Here's the drawing with two shaded views (mm, measured from the low corner). I have some questions. A direction names the side the tool comes from. Round coordinates to 2 decimals unless told otherwise and drop trailing zeros. Loops run counter-clockwise (first coordinate to the right, second up) from the corner with the lowest first, then second, coordinate; pieces in that order, holes last. Notation, with made-up numbers: (10, 26.25) - (38, 26.25) arc R28 cw to (38, 52.25) - close; hole circle Ø11 at (52, 64.25). An arc over 180 degrees is marked (long way). Answer as CSV lines item,"result".
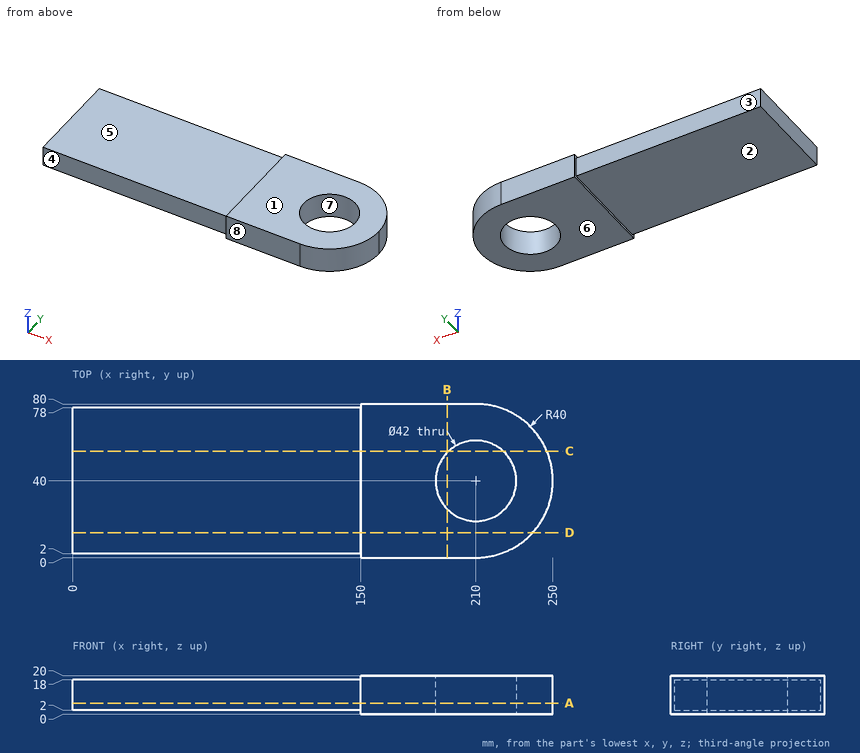
Q1. Imagine slicing it at D-D (y = 13). Write out the boundary of the cut face in (x, z).
Checks:
outline,"(0, 2) - (150, 2) - (150, 0) - (239.51, 0) - (239.51, 20) - (150, 20) - (150, 18) - (0, 18) - close"
Q2. Imagine slicing it at B-B (x = 195). Write out the boundary of the cut face in (y, z).
Checks:
outline,"(0, 0) - (25.3, 0) - (25.3, 20) - (0, 20) - close; (54.7, 0) - (80, 0) - (80, 20) - (54.7, 20) - close"
Q3. Imagine slicing it at C-C (y = 55.5). Write out the boundary of the cut face in (x, z), then the cut area to 3 significant figures.
Checks:
outline,"(0, 2) - (150, 2) - (150, 0) - (195.83, 0) - (195.83, 20) - (150, 20) - (150, 18) - (0, 18) - close; (224.17, 0) - (246.87, 0) - (246.87, 20) - (224.17, 20) - close"
area,"3,770 mm²"
Q4. We'd pull the mould along Y, two halves only. Please class the marked faces 6, 7 and 8: pulls with the +Y half, pulls with the -Y half, needs draft (parallel to the pull), parting line crosses it, or undercut.
Checks:
face 6,"needs draft"
face 7,"undercut"
face 8,"pulls with the -Y half"
Q5. If I drill on line 1 along Y through (x, z) = (210, 8); line 2 along Y through (x, z) = (145, 17.75); line 3 along Z through (x, y) = (142, 28.5), over which ranges is the centre line in solid material (lowest first)? Write a range as [from, to].
Checks:
line 1,"[0, 19], [61, 80]"
line 2,"[2, 78]"
line 3,"[2, 18]"
Q6. Imagine slicing it at A-A (z = 5.75). Write out the boundary of the cut face in (x, y).
Checks:
outline,"(0, 2) - (150, 2) - (150, 0) - (210, 0) arc R40 ccw to (210, 80) - (150, 80) - (150, 78) - (0, 78) - close; hole circle Ø42 at (210, 40)"
Q7. I'm going to push flat-ended pins straight in: pin 1 Ø5 at (x, z) = (93, 5.5) entering from -Y; pin 2 Ø8 at (y, z) = (52, 9.5) entering from +X; pin 3 Ø23 at (x, y) = (59, 43) entering from +Z. Where does each tip first touch, or does it pass through?
Checks:
pin 1,"y = 2"
pin 2,"x = 249.19"
pin 3,"z = 18"
Q8. On a 3-axis mill with a long thin cutter (end or side, diameter ignored), from which of +Z, -Z, +X, -X, +Y, -Y can I reach the whole of each face in a straight line? I mean the marked faces 1, 2, 3, 4 and 5. Say none if no direction works.
Checks:
face 1,"+Z, +X, -X, +Y, -Y"
face 2,"-Z, -X, +Y, -Y"
face 3,"+Z, -Z, -X, +Y"
face 4,"+Z, -Z, -X, -Y"
face 5,"+Z, -X, +Y, -Y"
